Part model, mm, in its own coordinate system. Face numbers are marked on the shaded views. A direction names the side the tool comes from. Round coordinates to 2 decimals unless told otherwise and drop trailing zeros. Loops run counter-clockwise (first coordinate to the right, second up) from the corner with the lowest first, then second, coordinate; pieces in that order, holes last. Notation, with made-up numbers: (-15.75, 28.5) - (32.25, 28.5) arc R32 cw to (32.25, 56.5) - close; hole circle Ø4 at (49, 48). An arc over 180 degrees is marked (long way). Put each result on its own line as item: value.
Autodesk Inventor part; units mm, degrees
ref_plane "YZ Plane" through (0, 0, 0) normal (1, 0, 0) x (0, 1, 0)
ref_plane "XZ Plane" through (0, 0, 0) normal (0, 1, 0) x (-1, 0, 0)
ref_plane "XY Plane" through (0, 0, 0) normal (0, 0, 1) x (1, 0, 0)
sketch "Sketch19" plane through (0, 0, 0) normal (1, 0, 0) x (0, 1, 0)
  line L0 (0, 0) -> (0, -22)
  line L1 (0, -22) -> (10.1375, -58.6184)
  line L2 (10.5, -61.2865) -> (10.5, -86.2865)
  line L3 (10.5, -86.2865) -> (17, -86.2865)
  line L4 (17, -86.2865) -> (17, -61.2865)
  line L5 (16.6375, -58.6184) -> (6.5, -22)
  line L6 (6.5, -22) -> (6.5, 0)
  line L7 (6.5, 0) -> (0, 0)
  arc A0 (10.5, -61.2865) -> (10.1375, -58.6184) centre (0.5, -61.2865) ccw
  arc A1 (17, -61.2865) -> (16.6375, -58.6184) centre (7, -61.2865) ccw
  point P0 (16.909, -59.9402)
  dimension "d79" = 10
  dimension "d80" = 10
  dimension "d82" = 6.5
  dimension "d83" = 10.5
  dimension "d84" = 25
  dimension "d85" = 22
  dimension "d86" = 37.9402
extrude "Extrusion7" add sketch "Sketch19" along normal blind 12
sketch "Sketch20" plane through (0, 6.5, 0) normal (0, 1, 0) x (1, 0, 0)
  circle A0 centre (6, 6) radius 6
  line L0 (0, 0) -> (12, 0)
  line L1 (0, 0) -> (12, 0)
  line L2 (0, 0) -> (0, 6)
  line L3 (0, 0) -> (0, 22)
  line L4 (12, 0) -> (12, 6)
  point P0 (6, 0)
  point P1 (6, 0)
  dimension "d89" = 12
extrude "Extrusion8" cut sketch "Sketch20" against normal blind 12 contours L4 L0 A0 | A0 L0 L2
sketch "Sketch21" plane through (0, 17, -61.2865) normal (0, 1, 0) x (1, 0, 0)
  circle A0 centre (6, 21) radius 4
  line L0 (0, 25) -> (12, 25)
  arc A1 (0, -55.2865) -> (12, -55.2865) centre (6, -55.2865) ccw
  line L1 (12, -39.2865) -> (12, -55.2865)
  line L2 (0, -39.2865) -> (12, -39.2865)
  line L3 (0, -39.2865) -> (0, -55.2865)
  line L4 (0, -39.2865) -> (2.0022, 21.1325)
  line L5 (12, -39.2865) -> (12, -2.6681)
  line L6 (12, -39.2865) -> (9.9978, 21.1325)
  line L7 (0, 25) -> (0, 0)
  line L8 (0, -39.2865) -> (0, 25)
  line L9 (0, 25) -> (6, 25)
  line L10 (6, 25) -> (12, 25)
  line L11 (12, 0) -> (12, 25)
  line L12 (12, 25) -> (12, -39.2865)
  point P0 (0, -61.2865)
  point P1 (12, 0)
  dimension "d93" = 8
extrude "Extrusion9" cut sketch "Sketch21" against normal up to surface (17 mm away) contours A0 L0 L11 L12 L5 L6 | L4 L8 L7 L0 A0
sketch "Sketch22" plane through (6, 6.5, -6) normal (0, 1, 0) x (1, 0, 0)
  arc A0 (-6, 0) -> (6, 0) centre (0, 0) ccw
  point P0 (-6, -6)
hole "Hole1" at (6, 6.5, -6) direction (0, -1, 0) diameter 10 end through all
sketch "Sketch23" plane through (6, 17, -82.2865) normal (0, 1, 0) x (1, 0, 0)
  arc A0 (3.9978, 0.1325) -> (-3.9978, 0.1325) centre (0, 0) ccw
  point P0 (-6, -82.2865)
hole "Hole2" at (6, 17, -82.2865) direction (0, -1, 0) diameter 5 end through all
fillet "Fillet1" radius 10 1 edges at (6, 6.5, -22)
properties part number "47A"
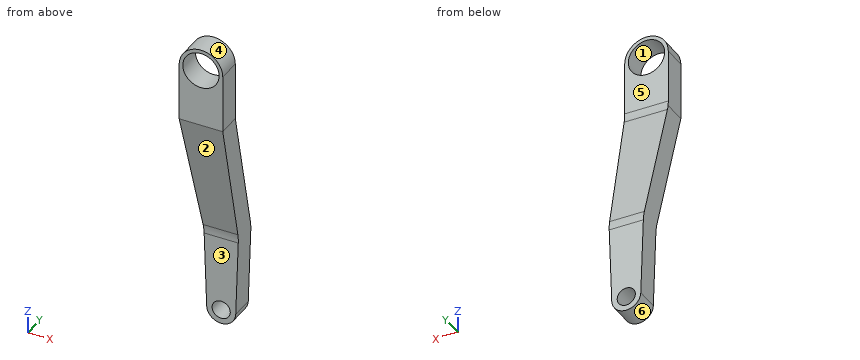
1. Pin check, flat tips, straight feed: P1, Ø1.5, axis at x = 7, y = 14, coming from the -Z side; P2, Ø1, axis at x = 8.5, z = -59, coming from the -Y side; P3, Ø4, axis at y = 8.5, z = -25.5, coming from the +X side. Stop position of each tip, or through.
A:
P1: stops at z = -86.28
P2: stops at y = 10.1
P3: stops at x = 11.93
2. Tool access for the marked faces 5 and 6: list every direction of +Z, -Z, +X, -X, +Y, -Y with a clear straight run to the whole face (end or side of a thin tool).
A:
face 5: +Z, +X, -X, +Y
face 6: -Z, +Y, -Y
3. Probe line 1 along Y through (x, z) = (8, -75); line 2 along Y through (x, z) = (9, -50.5); line 3 along X through (y, z) = (12.5, -64). List the from-to ranges inside material, lowest first. Write a range as [from, to].
A:
line 1: y = [10.5, 17]
line 2: y = [7.89, 14.39]
line 3: x = [1.39, 10.61]
4. Band-saw the part on A-A (x = 6). List the corners of the cut face in (y, z), plus the area to 3 significant figures.
A:
outline: (0, -22) - (10.14, -58.62) arc R10 cw to (10.5, -61.29) - (10.5, -79.79) - (17, -79.79) - (17, -61.29) arc R10 ccw to (16.64, -58.62) - (6.86, -23.31) arc R10 cw to (6.5, -20.64) - (6.5, -11) - (0, -11) - close; (0, -1) - (6.5, -1) - (6.5, 0) - (0, 0) - close; (10.5, -86.29) - (17, -86.29) - (17, -84.79) - (10.5, -84.79) - close
area: 463 mm²
5. Two-plate mould, pull along Z, no slides. Class the marked faces 1, 2, 3 and 4: pulls with the +Z half, pulls with the -Z half, needs draft (parallel to the pull), parting line crosses it, or undercut.
A:
face 1: undercut
face 2: pulls with the -Z half
face 3: needs draft
face 4: pulls with the +Z half
6. Band-saw the part on B-B (z = -8). List the corners of the cut face in (x, y), plus the area to 3 significant figures.
A:
outline: (0, 0) - (1.42, 0) - (1.42, 6.5) - (0, 6.5) - close; (10.58, 0) - (12, 0) - (12, 6.5) - (10.58, 6.5) - close
area: 18.4 mm²
7. Band-saw the part on D-D (z = -47). List the corners of the cut face in (x, y).
A:
outline: (0.83, 6.92) - (11.17, 6.92) - (11.17, 13.42) - (0.83, 13.42) - close
8. Band-saw the part on C-C (y = 2.5). List the corners of the cut face in (x, z), plus the area to 3 significant figures.
A:
outline: (0, -22) - (0.3, -31.03) - (11.7, -31.03) - (12, -22) - (12, -6) arc R6 ccw to (0, -6) - close; hole circle Ø10 at (6, -6)
area: 276 mm²
